Geometry: final body of the model. Coordinates: model frame, mm. Coordinates: 2 decimals unless noted, no trailing zeros. Loops run counter-clockwise (first coordinate to the right, second up) from the corner with the lowest first, then second, coordinate; pieces in that order, holes last. Notation, with made-up numbers: (44.5, 80) -> (54.5, 80) arc R13 ccw to (54.5, 102) -> close; hole circle Ø3 at (83.5, 27). An arc over 180 degrees is marked (long way). One line per item, written item: value. Start each with the question number.
Item 1: Section query A-A on z = 161. Return loops of the section in (x, y).
Item 2: Ray query, probe 1 along X at (y, z) = (0.5, 269); probe 2 along Y at (x, z) = (66.5, 6.35); probe 3 along Z at (x, y) = (5, 5.25). Return the intervals inside material, ascending. Write a range as from..to.
Item 3: Section query B-B on x = 28.5. Return loops of the section in (y, z), then the cut area to 3 significant figures.
Item 4: Contact query for flat-ended pins moving along their axis: pin 1 Ø7 at (y, z) = (6.35, 298.45) entering from +X; pin 2 Ø2 at (x, y) = (61.5, 6) entering from +Z; pin 3 Ø5 at (x, y) = (68, 9) entering from -Z; pin 4 Ø6.5 at (y, z) = (6, 24) entering from +X. Output: stop coordinate, or through.
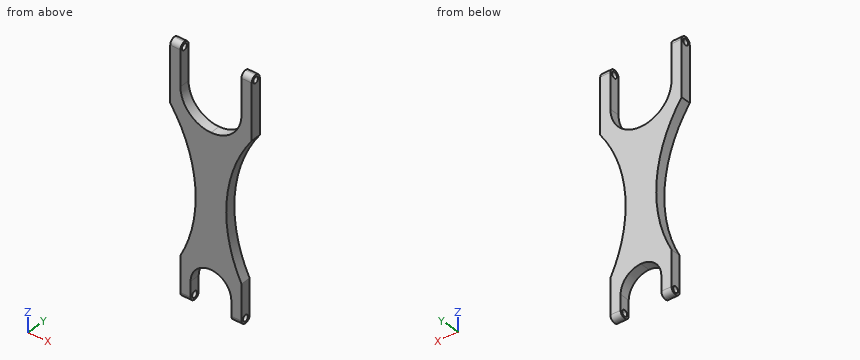
from build123d import *

# Parameters (mm, degrees)
BOSS_EXTRUDE1_DEPTH = 12.7
FILLET1_R           = 6.35
SKETCH2_R           = 3.81
CUT_EXTRUDE1_DEPTH  = 322.53831809
SKETCH3_R           = 3.81
CUT_EXTRUDE2_DEPTH  = 318.753898481


with BuildPart() as part:
    # Sketch1 → Boss-Extrude1 (new body)
    with BuildSketch(Plane(origin=(0, 0, 0), x_dir=(1, 0, 0), z_dir=(0, 1, 0))):
        with BuildLine():
            Line((0, 0), (12.7, 0))
            Line((12.7, 0), (12.7, -25.4))
            ThreePointArc((12.7, -25.4), (20.139487758, -43.360512242), (38.1, -50.8))
            ThreePointArc((38.1, -50.8), (56.060512242, -43.360512242), (63.5, -25.4))
            Line((63.5, -25.4), (63.5, 0))
            Line((63.5, 0), (76.2, 0))
            Line((76.2, 0), (76.2, -50.8))
            ThreePointArc((76.2, -50.8), (57.621017373, -141.480641616), (88.9, -228.6))
            Line((88.9, -228.6), (88.9, -304.8))
            Line((88.9, -304.8), (76.2, -304.8))
            Line((76.2, -304.8), (76.2, -254))
            ThreePointArc((76.2, -254), (65.040768363, -227.059231637), (38.1, -215.9))
            ThreePointArc((38.1, -215.9), (11.159231637, -227.059231637), (0, -254))
            Line((0, -254), (0, -304.8))
            Line((0, -304.8), (-12.7, -304.8))
            Line((-12.7, -304.8), (-12.7, -228.6))
            ThreePointArc((-12.7, -228.6), (18.578982627, -141.480641616), (0, -50.8))
            Line((0, -50.8), (0, 0))
        make_face()
    extrude(amount=BOSS_EXTRUDE1_DEPTH)

    # Fillet1
    fillet1_edges = [part.edges().sort_by_distance(p)[0] for p in [
        (69.85, 0, 0),
        (6.35, 0, 0),
        (69.85, 12.7, 0),
        (6.35, 12.7, 0),
        (-6.35, 0, 304.8),
        (-6.35, 12.7, 304.8),
        (82.55, 0, 304.8),
        (82.55, 12.7, 304.8),
    ]]
    fillet(fillet1_edges, radius=FILLET1_R - 0.0001)  # a hair under: the kernel refuses the full size

    # Sketch2 → Cut-Extrude1 (cut, through all)
    with BuildSketch(Plane(origin=(88.9, 0, 0), x_dir=(0, 0, -1), z_dir=(1, 0, 0))):
        with Locations((-298.45, 6.35)):
            Circle(SKETCH2_R)
    extrude(amount=-CUT_EXTRUDE1_DEPTH, mode=Mode.SUBTRACT)

    # Sketch3 → Cut-Extrude2 (cut, through all)
    with BuildSketch(Plane(origin=(76.2, 0, 0), x_dir=(0, 0, -1), z_dir=(1, 0, 0))):
        with Locations((-6.35, 6.35)):
            Circle(SKETCH3_R)
    extrude(amount=-CUT_EXTRUDE2_DEPTH, mode=Mode.SUBTRACT)


solid = part.part
Reply:
1. outline: (16.05, 0) -> (60.15, 0) -> (60.15, 12.7) -> (16.05, 12.7) -> close
2. probe 1: x = -12.7..0, 76.2..88.9
2. probe 2: y = 0..2.54, 10.16..12.7
2. probe 3: z = 0.1..2.7, 10..61.38, 197.15..235.13
3. outline: (0, 48.92) -> (12.7, 48.92) -> (12.7, 217.13) -> (0, 217.13) -> close
3. area: 2,140 mm²
4. pin 1: passes through
4. pin 2: stops at z = 224.74
4. pin 3: stops at z = 0
4. pin 4: stops at x = 76.2
